Source: CAD feature listing. Evaluate the final solid. Frame: model axes, mm. Round coordinates to 2 decimals unless told otherwise and drop trailing zeros. Order: outer loops, then holes, each group sorted by start corner. A loop starts at its lowest first (then second) coordinate and runs counter-clockwise, first axis right, second up.
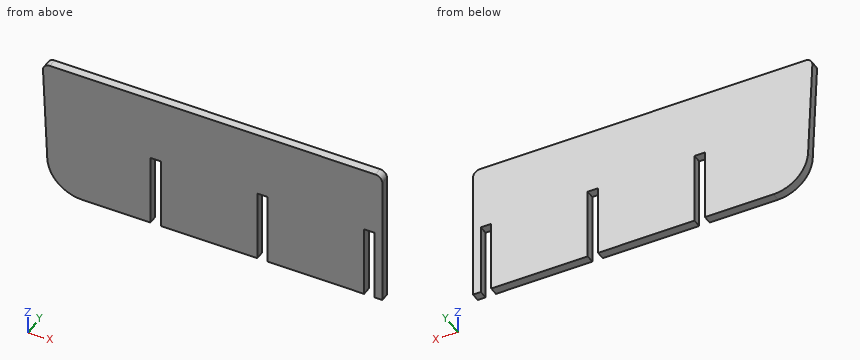
```python
from build123d import *

# Parameters (mm, degrees)
F1_DEPTH = 3.175
F2_R     = 25.4
F3_R     = 5.08


with BuildPart() as f1:
    # F0 (on Front) → F1 (new body, symmetric)
    with BuildSketch(Plane.XZ):
        Polygon((122.2375, 101.6), (-126.673452, 101.6), (-122.2375, 0), (-47.722367, 0), (-47.722367, 53.34), (-40.102367, 53.34), (-40.102367, 0), (30.585833, 0), (30.585833, 53.34), (38.205833, 53.34), (38.205833, 0), (108.9025, 0), (108.9025, 53.34), (116.5225, 53.34), (116.5225, 0), (122.2375, 0), align=None)
    extrude(amount=F1_DEPTH, both=True)

    # F2
    f2_edges = [f1.edges().sort_by_distance(p)[0] for p in [
        (-122.2375, 0, 0),
    ]]
    fillet(f2_edges, radius=F2_R)

    # F3
    f3_edges = [f1.edges().sort_by_distance(p)[0] for p in [
        (-126.673452, 0, 101.6),
        (122.2375, 0, 101.6),
    ]]
    fillet(f3_edges, radius=F3_R)


solid = f1.part
```
1. First-contact query: pin 1 (1.9 mm diameter, centred on y = -1, z = 27, fed in from -X); pin 2 (1.9 mm diameter, centred on x = 111.5, y = 1, fed in from -Z); pin 3 (3 mm diameter, centred on y = 0.5, z = 15, fed in from -X). Flat tips, straight axial feed; report the tip coordinate or a pass-through.
2. Line query: line 1 along X through (y, z) = (-1, 22); line 2 along X through (y, z) = (-0.5, 8); line 3 along Z through (x, y) = (-45, -0.25). Output: solid intervals per line, ascending.
3. Section A-A on z = 7. Return loops of the section in (x, y) (1 decimal).
4. Section B-B on y = 0.5. Return loops of the section in (x, z), plus the area to 3 significant figures.
5. Section C-C on z = 30.5. Return loops of the section in (x, y) (1 decimal), plus the area to 3 significant figures.
Result:
1. pin 1: stops at x = -123.46
1. pin 2: stops at z = 53.34
1. pin 3: stops at x = -121.71
2. line 1: x = -123.09 to -47.72, -40.1 to 30.59, 38.21 to 108.9, 116.52 to 122.24
2. line 2: x = -116.43 to -47.72, -40.1 to 30.59, 38.21 to 108.9, 116.52 to 122.24
2. line 3: z = 53.34 to 101.6
3. outline: (-115.4, -3.2) - (-47.7, -3.2) - (-47.7, 3.2) - (-115.4, 3.2) - close; (-40.1, -3.2) - (30.6, -3.2) - (30.6, 3.2) - (-40.1, 3.2) - close; (38.2, -3.2) - (108.9, -3.2) - (108.9, 3.2) - (38.2, 3.2) - close; (116.5, -3.2) - (122.2, -3.2) - (122.2, 3.2) - (116.5, 3.2) - close
4. outline: (-126.44, 96.3) - (-123.3, 24.29) arc R25.4 ccw to (-97.92, 0) - (-47.72, 0) - (-47.72, 53.34) - (-40.1, 53.34) - (-40.1, 0) - (30.59, 0) - (30.59, 53.34) - (38.21, 53.34) - (38.21, 0) - (108.9, 0) - (108.9, 53.34) - (116.52, 53.34) - (116.52, 0) - (122.24, 0) - (122.24, 96.52) arc R5.08 ccw to (117.16, 101.6) - (-121.37, 101.6) arc R5.08 ccw to start
4. area: 23,700 mm2
5. outline: (-123.6, -3.2) - (-47.7, -3.2) - (-47.7, 3.2) - (-123.6, 3.2) - close; (-40.1, -3.2) - (30.6, -3.2) - (30.6, 3.2) - (-40.1, 3.2) - close; (38.2, -3.2) - (108.9, -3.2) - (108.9, 3.2) - (38.2, 3.2) - close; (116.5, -3.2) - (122.2, -3.2) - (122.2, 3.2) - (116.5, 3.2) - close
5. area: 1,420 mm2
